Here's how the part is built. I have some questions about the finished solid (model axes, mm). Face numbers are marked on the shaded views. A direction names the side the tool comes from. Coordinates: 2 decimals unless noted, no trailing zeros. Write each loop counter-clockwise with the first axis right and the second up, starting at its lowest first coordinate (ties: lowest second). Pieces come first, ordered by that corner, then holes. Notation, with made-up numbers: (42, -30) -> (79, -30) arc R28 cw to (79, -6) -> close; hole circle Ø3 at (26, 70). An arc over 180 degrees is marked (long way). Put each result on its own line as item: value. Start each with the question number.
Item 1: If we mould it in two halves opening along Y, with no side actions, what happens to the marked faces 1 and 2? For each: released by +Y, released by -Y, zero draft, split by the parting line, or undercut.
Item 2: I want a section at A-A, the plane x = 126. List the corners of the cut face in (y, z) for me.
Item 3: On a 3-axis mill with a long thin cutter (end or side, diameter ignored), from which of +Z, -Z, +X, -X, +Y, -Y can I reach the whole of each face in a straight line? I mean the marked faces 3, 4 and 5. Say none if no direction works.
Item 4: For pin 1 (4.5 mm diameter, centred on x = -105, y = -73, fed in from +Z); pin 2 (6 mm diameter, centred on x = -1, y = -114.5, fed in from +Z); pin 3 (1.5 mm diameter, centred on y = 27.5, z = 14.5, fed in from -X); pin 4 (8 mm diameter, centred on y = 87.5, z = 24.5, fed in from -X), each with a flat end and sliding along its axis, tell me the tip position at first contact or that it passes through.
Item 5: I need wall thicknesses on line 1 (X direction, y = -65, z = 4.75); line 2 (Y direction, x = -113.5, z = 22); line 3 (X direction, y = 110, z = 14.5). Which ranges of each line are inside material? Lowest first, please. Write a range as [from, to].
from build123d import *

# Parameters (mm, degrees)
SKETCH_1_W                = 300
SKETCH_1_H                = 250
EXTRUDE_1_DEPTH           = 30
SKETCH_2_W                = 180
SKETCH_2_H                = 175
CUT_EXTRUDE_1_DEPTH       = 15
FILLET_1_R                = 10
HOLE_WIZARD_1_D           = 9
HOLE_WIZARD_1_CBORE_D     = 15
HOLE_WIZARD_1_CBORE_DEPTH = 9
CHAMFER_1_SIZE            = 3
SKETCH_6_R                = 17.5
CUT_EXTRUDE_2_DEPTH       = 198.547462651
CHAMFER_2_SIZE            = 2
HOLE_WIZARD_M6_1_D        = 5
HOLE_WIZARD_M6_1_DEPTH    = 15
HOLE_WIZARD_M6_1_TIP      = 1.502151548
HOLE_WIZARD_M6_2_D        = 5
HOLE_WIZARD_M5_1_D        = 4.2
HOLE_WIZARD_M5_1_DEPTH    = 12.4
HOLE_WIZARD_M5_1_TIP      = 1.2618073
HOLE_WIZARD_M2_1_D        = 1.6
HOLE_WIZARD_M2_1_DEPTH    = 9.2
HOLE_WIZARD_M2_1_TIP      = 0.480688495
HOLE_WIZARD_M3_1_D        = 2.5
HOLE_WIZARD_M3_1_DEPTH    = 9.5
HOLE_WIZARD_M3_1_TIP      = 0.751075774
SKETCH_21_R               = 10.25
CUT_EXTRUDE_3_DEPTH       = 8
HOLE_WIZARD_M5_2_D        = 4.2
HOLE_WIZARD_M5_2_DEPTH    = 12.4
HOLE_WIZARD_M5_2_TIP      = 1.2618073


with BuildPart() as part:
    # 草图1 → 凸台-拉伸1 (new body)
    with BuildSketch(Plane.XY):
        Rectangle(SKETCH_1_W, SKETCH_1_H)
    extrude(amount=EXTRUDE_1_DEPTH)

    # 草图2 → 切除-拉伸1 (cut)
    with BuildSketch(Plane.XY.offset(30)):
        with Locations((-150, 0)):
            Rectangle(SKETCH_2_W, SKETCH_2_H)
        with Locations((150, 0)):
            Rectangle(SKETCH_2_W, SKETCH_2_H)
    extrude(amount=-CUT_EXTRUDE_1_DEPTH, mode=Mode.SUBTRACT)

    # 圆角1
    fillet_1_edges = [part.edges().sort_by_distance(p)[0] for p in [
        (-150, -87.5, 22.5),
        (-60, -87.5, 22.5),
        (-150, 87.5, 22.5),
        (-60, 87.5, 22.5),
        (150, 87.5, 22.5),
        (60, 87.5, 22.5),
        (150, -87.5, 22.5),
        (60, -87.5, 22.5),
        (150, -125, 15),
        (-150, -125, 15),
        (-150, 125, 15),
        (150, 125, 15),
    ]]
    fillet(fillet_1_edges, radius=FILLET_1_R)

    # 打孔尺寸(%根据)内六角圆柱头螺钉的类型1 (through all)
    with Locations(Plane.XY.offset(30)):
        with Locations((-20, 20), (20, 20), (20, -20), (-20, -20)):
            CounterBoreHole(HOLE_WIZARD_1_D / 2, HOLE_WIZARD_1_CBORE_D / 2, HOLE_WIZARD_1_CBORE_DEPTH)

    # 倒角1
    chamfer_1_edges = [part.edges().sort_by_distance(p)[0] for p in [
        (-150, 0, 15),
        (150, 0, 15),
        (0, -125, 0),
        (0, -125, 30),
        (150, 0, 0),
        (-150, 0, 0),
        (0, 125, 0),
        (-147.071067812, 122.071067812, 0),
        (147.071067812, 122.071067812, 0),
        (147.071067812, -122.071067812, 0),
        (-147.071067812, -122.071067812, 0),
        (-150, -106.25, 30),
        (-150, 106.25, 30),
        (-105, -87.5, 30),
        (150, -106.25, 30),
        (105, -87.5, 30),
        (60, 0, 30),
        (105, 87.5, 30),
        (150, 106.25, 30),
        (0, 125, 30),
        (-105, 87.5, 30),
        (-60, 0, 30),
        (-147.071067812, 90.428932188, 30),
        (-147.071067812, -90.428932188, 30),
        (147.071067812, 90.428932188, 30),
        (147.071067812, -90.428932188, 30),
        (-147.071067812, 122.071067812, 30),
        (147.071067812, 122.071067812, 30),
        (147.071067812, -122.071067812, 30),
        (-147.071067812, -122.071067812, 30),
        (62.928932188, -84.571067812, 30),
        (62.928932188, 84.571067812, 30),
        (-62.928932188, -84.571067812, 30),
        (-62.928932188, 84.571067812, 30),
    ]]
    chamfer(chamfer_1_edges, length=CHAMFER_1_SIZE)

    # 草图6 → 切除-拉伸2 (cut, through all)
    with BuildSketch(Plane.XY.offset(30)):
        Circle(SKETCH_6_R)
    extrude(amount=-CUT_EXTRUDE_2_DEPTH, mode=Mode.SUBTRACT)

    # 倒角2
    chamfer_2_edges = [part.edges().sort_by_distance(p)[0] for p in [
        (-17.5, 0, 0),
        (-17.5, 0, 30),
    ]]
    chamfer(chamfer_2_edges, length=CHAMFER_2_SIZE)

    # M6 螺纹孔1
    with Locations(Plane(origin=(0, 0, 0), x_dir=(-1, 0, 0), z_dir=(0, 0, -1))):
        with Locations((-20, 95), (20, -95), (-20, -95), (-20, -65), (20, -65), (65, -20), (95, -20), (95, 20), (65, 20), (-65, -20), (-95, -20), (-95, 20), (-65, 20), (20, 65), (20, 95), (-20, 65)):
            Hole(HOLE_WIZARD_M6_1_D / 2, depth=HOLE_WIZARD_M6_1_DEPTH)
            with Locations((0, 0, -(HOLE_WIZARD_M6_1_DEPTH + HOLE_WIZARD_M6_1_TIP / 2))):  # 118° drill point
                Cone(0, HOLE_WIZARD_M6_1_D / 2, HOLE_WIZARD_M6_1_TIP, mode=Mode.SUBTRACT)

    # M6 螺纹孔2 (through all)
    with Locations(Plane.XY.offset(15)):
        with Locations((-105, 73), (-105, -73), (105, 73), (105, -73)):
            Hole(HOLE_WIZARD_M6_2_D / 2)

    # M5 螺纹孔1
    with Locations(Plane(origin=(0, -125, 0), x_dir=(-1, 0, 0), z_dir=(0, -1, 0))):
        with Locations((65, -15), (-65, -15)):
            Hole(HOLE_WIZARD_M5_1_D / 2, depth=HOLE_WIZARD_M5_1_DEPTH)
            with Locations((0, 0, -(HOLE_WIZARD_M5_1_DEPTH + HOLE_WIZARD_M5_1_TIP / 2))):  # 118° drill point
                Cone(0, HOLE_WIZARD_M5_1_D / 2, HOLE_WIZARD_M5_1_TIP, mode=Mode.SUBTRACT)

    # M2 螺纹孔1
    with Locations(Plane.XY.offset(30)):
        with Locations((11.691342951, 58.75), (0, 79), (-11.691342951, 58.75)):
            Hole(HOLE_WIZARD_M2_1_D / 2, depth=HOLE_WIZARD_M2_1_DEPTH)
            with Locations((0, 0, -(HOLE_WIZARD_M2_1_DEPTH + HOLE_WIZARD_M2_1_TIP / 2))):  # 118° drill point
                Cone(0, HOLE_WIZARD_M2_1_D / 2, HOLE_WIZARD_M2_1_TIP, mode=Mode.SUBTRACT)

    # M3 螺纹孔1
    with Locations(Plane.XY.offset(30)):
        with Locations((-42.5, 0), (42.5, 0)):
            Hole(HOLE_WIZARD_M3_1_D / 2, depth=HOLE_WIZARD_M3_1_DEPTH)
            with Locations((0, 0, -(HOLE_WIZARD_M3_1_DEPTH + HOLE_WIZARD_M3_1_TIP / 2))):  # 118° drill point
                Cone(0, HOLE_WIZARD_M3_1_D / 2, HOLE_WIZARD_M3_1_TIP, mode=Mode.SUBTRACT)

    # 草图21 → 切除-拉伸3 (cut)
    with BuildSketch(Plane.XY.offset(30)):
        with Locations((0, 110)):
            Circle(SKETCH_21_R)
        with Locations((0, -110)):
            Circle(SKETCH_21_R)
    extrude(amount=-CUT_EXTRUDE_3_DEPTH, mode=Mode.SUBTRACT)

    # M5 螺纹孔2
    with Locations(Plane.XY.offset(22)):
        with Locations((0, -110), (0, 110)):
            Hole(HOLE_WIZARD_M5_2_D / 2, depth=HOLE_WIZARD_M5_2_DEPTH)
            with Locations((0, 0, -(HOLE_WIZARD_M5_2_DEPTH + HOLE_WIZARD_M5_2_TIP / 2))):  # 118° drill point
                Cone(0, HOLE_WIZARD_M5_2_D / 2, HOLE_WIZARD_M5_2_TIP, mode=Mode.SUBTRACT)


solid = part.part
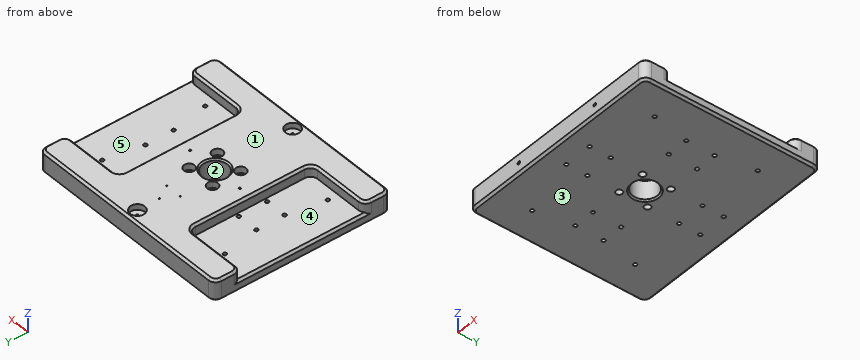
Calculated:
1. face 1: zero draft
1. face 2: undercut
2. outline: (-125, 3) -> (-122, 0) -> (122, 0) -> (125, 3) -> (125, 27) -> (122, 30) -> (90.5, 30) -> (87.5, 27) -> (87.5, 15) -> (-87.5, 15) -> (-87.5, 27) -> (-90.5, 30) -> (-122, 30) -> (-125, 27) -> close
3. face 3: -Z, +X, -X, +Y, -Y
3. face 4: +Z, -X
3. face 5: +Z, +X
4. pin 1: passes through
4. pin 2: stops at z = 22
4. pin 3: stops at x = -148.25
4. pin 4: stops at x = -148
5. line 1: x = [-150, -22.5], [-17.5, 17.5], [22.5, 150]
5. line 2: y = [-125, -87.5], [87.5, 125]
5. line 3: x = [-150, -2.1], [2.1, 150]
